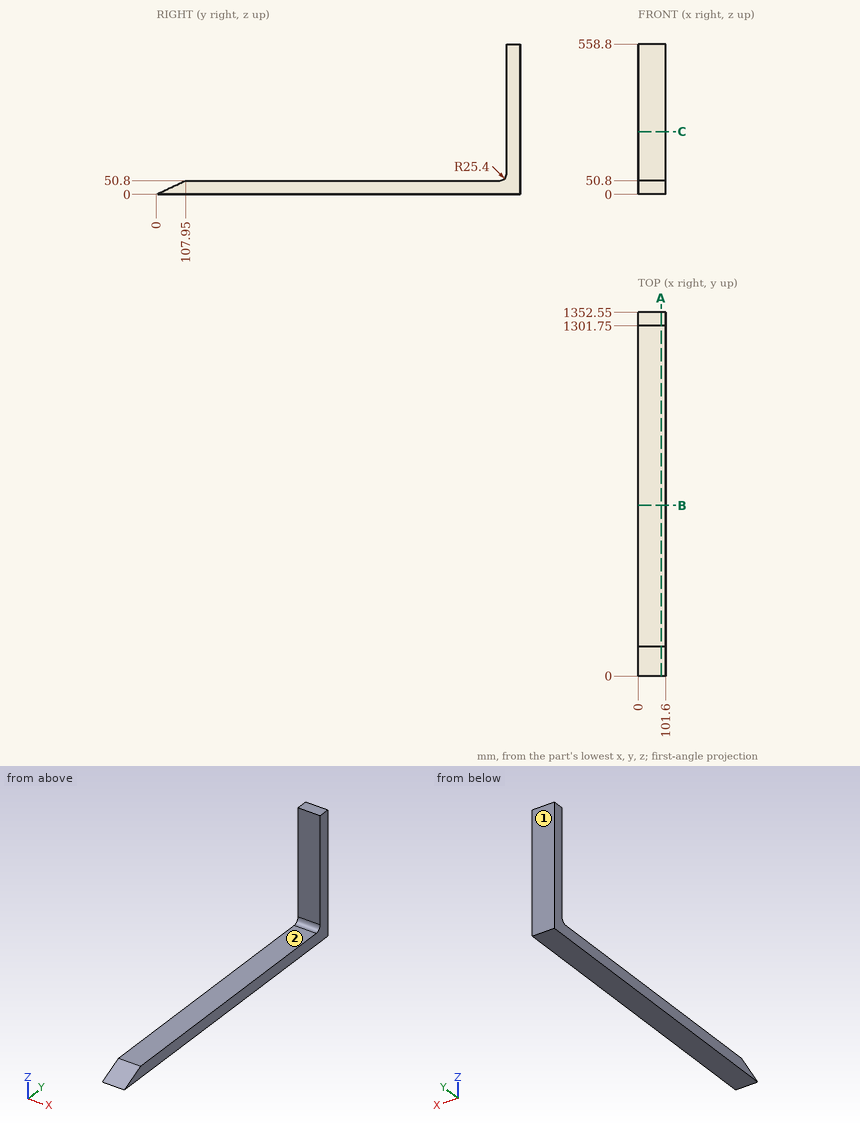
Study the drawing (mm; zero at the part's minimum x, y, z) and answer. A direction names the side the tool comes from. Round coordinates to 2 decimals unless told otherwise and drop trailing zeros. Write each loop counter-clockwise with the first axis right and the second up, starting at its lowest first coordinate (ties: lowest second). Pieces come first, ordered by that corner, then holes.
1) A cutting plane is placed at A-A (x = 85). Give the vertices of the cut face in (y, z).
2) A cutting plane is placed at C-C (z = 233). Give the vertices of the cut face in (x, y).
3) A tool of negligible diameter and unlimited length cuts with its end or side. For the marked faces 1 and 2, from which of +Z, -Z, +X, -X, +Y, -Y can it reach the whole face along a straight path? Write none if from no direction.
4) Given pin 1 Ø6 at (x, z) = (78, 194.5) entering from -Y; pin 2 Ø3 at (x, y) = (74.5, 1152) entering from -Z; pin 3 Ø3 at (x, y) = (13.5, 584) entering from +Z, each flat-ended and moving along its own axis, determine where each tip first touches the part or whether it passes through.
5) A cutting plane is placed at B-B (y = 634.5). Give the vertices of the cut face in (x, z), plus the area to 3 significant figures.
6) Straight lines are drawn through the part: line 1 (Z direction, x = 80.5, y = 1106.5); line 2 (Y direction, x = 32, z = 394.5); line 3 (Z direction, x = 13, y = 87.5). For each, find the intervals that lie inside material, in ascending order.
Completed:
1. outline: (0, 0) - (1352.55, 0) - (1352.55, 558.8) - (1301.75, 558.8) - (1301.75, 76.2) arc R25.4 cw to (1276.35, 50.8) - (107.95, 50.8) - close
2. outline: (0, 1301.75) - (101.6, 1301.75) - (101.6, 1352.55) - (0, 1352.55) - close
3. face 1: +Z, -Z, +X, -X, +Y
3. face 2: +Z, +X, -X, -Y
4. pin 1: stops at y = 1301.75
4. pin 2: stops at z = 0
4. pin 3: stops at z = 50.8
5. outline: (0, 0) - (101.6, 0) - (101.6, 50.8) - (0, 50.8) - close
5. area: 5,160 mm2
6. line 1: z = 0 to 50.8
6. line 2: y = 1301.75 to 1352.55
6. line 3: z = 0 to 41.18
